Source: CAD feature listing. Evaluate the final solid. Frame: model axes, mm. A direction names the side the tool comes from. Coordinates: 2 decimals unless noted, no trailing zeros. Loops run counter-clockwise (first coordinate to the right, second up) from the corner with the lowest first, then second, coordinate; pieces in that order, holes last.
Item 1: Section query A-A, the plane y = -5.75. Return the cut outline in (x, z), then the cut area to 3 significant figures.
Item 2: Section query C-C, the plane z = -7.25. Return the cut outline in (x, y).
Item 3: Pin query (flat end, axial travel): pin 1 Ø12 at (x, z) = (-3.5, -8.5) entering from +Y; pin 2 Ø4 at (x, y) = (-23, -7.5) entering from -Z; pin 3 Ø4 at (y, z) = (-9, 8) entering from +X. Return the tip coordinate at first contact, or that it passes through.
Item 4: Section query B-B, the plane x = -48.5. Return the cut outline in (y, z).
Item 5: Line query: probe 1 along Z at (x, y) = (-30.5, -5.25); probe 2 along X at (y, z) = (-11.25, 0.25); probe 3 along Z at (x, y) = (0.5, -5.25). Output: solid intervals per line, ascending.
Item 6: Reachability of faces 1 (the flat face through (-38, -6, 12.7)), 2 (the flat face through (-40, -6, -12.25)) from +Z, -Z, +X, -X, +Y, -Y: full face, straight path, thin tool, end or side. Return the list, or none.
```python
from build123d import *

# Parameters (mm, degrees)
F1_DEPTH = 12.7


with BuildPart() as f1:
    # F0 (on Front) → F1 (new body)
    with BuildSketch(Plane.XZ):
        with BuildLine():
            ThreePointArc((-3.351711, -12.249736), (-12.586931, 1.69091), (0, 12.7))
            Line((0, 12.7), (-76.620914, 12.7))
            Line((-76.620914, 12.7), (-76.620914, -12.249736))
            Line((-76.620914, -12.249736), (-3.351711, -12.249736))
        make_face()
        with BuildLine():
            Line((0, -12.249736), (0, 12.7))
            ThreePointArc((0, 12.7), (-12.586931, 1.69091), (-3.351711, -12.249736))
            Line((-3.351711, -12.249736), (0, -12.249736))
        make_face()
        with BuildLine():
            ThreePointArc((-3.351711, -12.249736), (7.70465, -10.095958), (12.7, 0))
            ThreePointArc((12.7, 0), (8.980256, 8.980256), (0, 12.7))
            Line((0, 12.7), (0, -12.249736))
            Line((0, -12.249736), (-3.351711, -12.249736))
        make_face()
    extrude(amount=F1_DEPTH)


solid = f1.part
```
Verdict:
1. outline: (-76.62, -12.25) - (-3.35, -12.25) arc R12.7 ccw (long way) to (0, 12.7) - (-76.62, 12.7) - close
1. area: 2,170 mm2
2. outline: (-76.62, -12.7) - (10.43, -12.7) - (10.43, 0) - (-76.62, 0) - close
3. pin 1: stops at y = 0
3. pin 2: stops at z = -12.25
3. pin 3: stops at x = 11.19
4. outline: (-12.7, -12.25) - (0, -12.25) - (0, 12.7) - (-12.7, 12.7) - close
5. probe 1: z = -12.25 to 12.7
5. probe 2: x = -76.62 to 12.7
5. probe 3: z = -12.69 to 12.69
6. face 1: +Z, +X, -X, +Y, -Y
6. face 2: -Z, -X, +Y, -Y
